from build123d import *

# Parameters (mm, degrees)
F0_W     = 38.1
F0_H     = 38.1
F0_R     = 6.58852
F1_DEPTH = 50.8


with BuildPart() as f1:
    # F0 (on Front) → F1 (new body)
    with BuildSketch(Plane.XZ):
        with Locations((19.05, 19.05)):
            Rectangle(F0_W, F0_H)
        with Locations((19.05, 19.05)):
            Circle(F0_R, mode=Mode.SUBTRACT)
        Polygon((-12.380896, 38.1), (0, 38.1), (38.1, 38.1), (50.480896, 38.1), (19.05, 69.530896), align=None)
        with Locations((19.05, 19.05)):
            Circle(F0_R)
    extrude(amount=F1_DEPTH)


solid = f1.part
CAD build for the part. Positions are in the model's coordinates, mm. A direction names the side the tool comes from. Give positions to 0.01 mm unless a question says otherwise; leave off trailing zeros. Loops run counter-clockwise (first coordinate to the right, second up) from the corner with the lowest first, then second, coordinate; pieces in that order, holes last. Notation, with made-up numbers: M 15,5 L 29,5 A4 cw 29,11 Z; hole C -18.75,58 d5. An arc over 180 degrees is marked long. Write each question's results on one line, items separated by ' | '.
Q1. Band-saw the part on B-B on z = 31.5. Write the cut outline in (x, y), and give its area (3 significant figures).
Geometry check:
outline: M 0,-50.8 L 38.1,-50.8 L 38.1,0 L 0,0 Z | area: 1,940 mm²
Q2. Band-saw the part on A-A on y = -22. Write the cut outline in (x, z), and give its area (3 significant figures).
Geometry check:
outline: M -12.38,38.1 L 0,38.1 L 0,0 L 38.1,0 L 38.1,38.1 L 50.48,38.1 L 19.05,69.53 Z | area: 2,440 mm²
Q3. Probe probe 1 along X at (y, z) = (-21, 29); probe 2 along X at (y, z) = (-14, 47); probe 3 along Z at (x, y) = (20, -22). List the from-to ranges inside material, lowest first.
Geometry check:
probe 1: x = 0 to 38.1 | probe 2: x = -3.48 to 41.58 | probe 3: z = 0 to 68.58
Q4. Flat gauge pins, fed straight in: P1, Ø10, axis at x = -6, y = -34, coming from the -Z side; P2, Ø5, axis at y = -20, z = 41.5, coming from the +X side; P3, Ø2, axis at y = -26.5, z = 14.5, coming from the -X side. Where does each tip first touch, or does it go through?
Geometry check:
P1: stops at z = 38.1 | P2: stops at x = 49.58 | P3: stops at x = 0
Q5. Which spindle directions (+Z, -Z, +X, -X, +Y, -Y) get a long thin tool onto all of the face, cutting with end or side? Do faces 1 (the face through (19, -50.8, 35)), 2 (the face through (0, -25, 19)), 3 (the face through (44, -25, 38.1)). Say none if no direction does.
Geometry check:
face 1: +Z, -Z, +X, -X, -Y | face 2: -Z, -X, +Y, -Y | face 3: -Z, +X, +Y, -Y
Q6. Band-saw the part on C-C on x = 43.5. Write the cut outline in (y, z), and give its area (3 significant figures).
Geometry check:
outline: M -50.8,38.1 L 0,38.1 L 0,45.08 L -50.8,45.08 Z | area: 355 mm²
